Read the model definition and answer for the solid it produces. Units are mm, in the model's axes. A direction names the side the tool comes from. Coordinates: 2 decimals unless noted, no trailing zeros. Order: outer loops, then holes, each group sorted by start corner. A loop starts at its lowest first (then second) coordinate and runs counter-clockwise, first axis right, second up. Notation, with made-up numbers: M 26,-30.5 L 34,-30.5 A32 ccw 34,1.5 Z; hole C -33,64 d9. An arc over 180 degrees is marked long. One line per question, with ' | ' between items. Start each with the question number.
1) Find section C-C, the plane y = 8.75. Write down the section's boundary in (x, z) (3 decimals), plus the area to 3 significant figures.
2) Find section B-B, the plane z = -1.5. Write down the section's boundary in (x, y), plus the area to 3 significant figures.
3) The mould has two halves that part along X. Classify faces 1 (the face through (157.096, -0.067, -1.565)), 2 (the face through (-3, 6, -3.175)): +X half, -X half, draft (parallel to the pull), parting line (faces both ways), or undercut.
4) Find section A-A, the plane x = -124.5. Write down the section's boundary in (y, z) (1 decimal), plus the area to 3 significant figures.
5) A tool of negligible diameter and unlimited length cuts with its end or side. For faces 3 (the face through (2, 0, 0)), 4 (the face through (-3, 0, 3.175)), from which of +Z, -Z, +X, -X, +Y, -Y can it reach the whole face along a straight path? Write none if from no direction.
6) Consider probe 1 along Y at (x, z) = (-79.5, -3); probe 2 along Z at (x, y) = (76, 3) (3 decimals); probe 3 along X at (y, z) = (-0.75, 2.5). Determine where each line is inside the solid, lowest interval first.
from build123d import *

# Parameters (mm, degrees)
F1_DEPTH = 3.175
F2_W     = 9.525
F2_H     = 3.175
F3_DEPTH = 152.4
F5_DEPTH = 9.525


# Not quite as in the source:
# - a length typed as a fraction of an inch, garbled in the dataset ("3 / 203.2 mm" for 3/8 in), is restored
# - a feature names something its author has since deleted; it is built from what else it names


with BuildPart() as f1:
    # F0 (on Top) → F1 (new body, symmetric)
    with BuildSketch(Plane.XY):
        with BuildLine():
            Line((-152.4, 12.7), (-177.8, 12.7))
            ThreePointArc((-177.8, 12.7), (-186.780256, 8.980256), (-190.5, 0))
            ThreePointArc((-190.5, 0), (-186.780256, -8.980256), (-177.8, -12.7))
            Line((-177.8, -12.7), (-152.4, -12.7))
            Line((-152.4, -12.7), (152.4, -12.7))
            Line((152.4, -12.7), (177.8, -12.7))
            ThreePointArc((177.8, -12.7), (186.780256, -8.980256), (190.5, 0))
            ThreePointArc((190.5, 0), (186.780256, 8.980256), (177.8, 12.7))
            Line((177.8, 12.7), (152.4, 12.7))
            Line((152.4, 12.7), (-152.4, 12.7))
        make_face()
    extrude(amount=F1_DEPTH, both=True)

    # F2 (on Right) → F3 (cut, symmetric)
    with BuildSketch(Plane.YZ):
        with Locations((0, -1.5875)):
            Rectangle(F2_W, F2_H)
    extrude(amount=F3_DEPTH, both=True, mode=Mode.SUBTRACT)

    # F4 (on face) → F5 (cut)
    with BuildSketch(Plane(origin=(0, -4.7625, 0), x_dir=(-1, 0, 0), z_dir=(0, 1, 0))):
        Polygon((161.925, -3.175), (152.4, 0), (152.4, -3.175), align=None)
        Polygon((-152.4, -3.175), (-152.4, 0), (-161.925, -3.175), align=None)
    extrude(amount=F5_DEPTH, mode=Mode.SUBTRACT)


solid = f1.part
Report:
1) outline: M -187.005,-3.175 L 187.005,-3.175 L 187.005,3.175 L -187.005,3.175 Z | area: 2,370 mm^2
2) outline: M -177.8,-12.7 L 177.8,-12.7 A12.7 ccw 177.8,12.7 L -177.8,12.7 A12.7 ccw Z; hole M -156.9,-4.76 L 156.9,-4.76 L 156.9,4.76 L -156.9,4.76 Z | area: 6,550 mm^2
3) face 1: undercut | face 2: draft
4) outline: M -12.7,-3.2 L -4.8,-3.2 L -4.8,0 L 4.8,0 L 4.8,-3.2 L 12.7,-3.2 L 12.7,3.2 L -12.7,3.2 Z | area: 131 mm^2
5) face 3: -Z | face 4: +Z, +X, -X, +Y, -Y
6) probe 1: y = -12.7 to -4.76, 4.76 to 12.7 | probe 2: z = 0 to 3.175 | probe 3: x = -190.48 to 190.48
